from build123d import *

# Parameters (mm, degrees)
BOSS_EXTRUDE1_DEPTH = 2
BOSS_EXTRUDE2_DEPTH = 5
CHAMFER1_SIZE       = 0.2


with BuildPart() as part:
    # Sketch1 → Boss-Extrude1 (new body)
    with BuildSketch(Plane(origin=(0, 0, 0), x_dir=(1, 0, 0), z_dir=(0, 1, 0))):
        with BuildLine():
            Line((60, 26), (30, 26))
            ThreePointArc((30, 26), (26, 30), (30, 34))
            Line((30, 34), (60, 34))
            Line((60, 34), (60, 60))
            Line((60, 60), (0, 60))
            Line((0, 60), (0, 0))
            Line((0, 0), (60, 0))
            Line((60, 0), (60, 26))
        make_face()
    extrude(amount=BOSS_EXTRUDE1_DEPTH)

    # Sketch2 → Boss-Extrude2 (add)
    with BuildSketch(Plane.XZ):
        Polygon((60, -12), (60, -10), (10, -10), (10, -60), (12, -60), (12, -12), align=None)
        Polygon((60, -2), (60, 0), (0, 0), (0, -60), (2, -60), (2, -10), (2, -2), (10, -2), align=None)
    extrude(amount=BOSS_EXTRUDE2_DEPTH)

    # Chamfer1
    chamfer1_edges = [part.edges().sort_by_distance(p)[0] for p in [
        (35, -5, -10),
        (10, -5, -35),
        (11, -5, -60),
        (12, -5, -36),
        (36, -5, -12),
        (60, -5, -11),
        (2, -5, -31),
        (31, -5, -2),
        (60, -5, -1),
        (30, -5, 0),
        (0, -5, -30),
        (1, -5, -60),
    ]]
    chamfer(chamfer1_edges, length=CHAMFER1_SIZE)


solid = part.part
Source: CAD feature listing. Evaluate the final solid. Frame: model axes, mm. A direction names the side the tool comes from. Round coordinates to 2 decimals unless told otherwise and drop trailing zeros. Loops run counter-clockwise (first coordinate to the right, second up) from the corner with the lowest first, then second, coordinate; pieces in that order, holes last. Notation, with made-up numbers: (-31.75, 79) -> (1.25, 79) arc R32 cw to (1.25, 108) -> close; hole circle Ø1 at (20.25, -1). An arc over 180 degrees is marked (long way). Answer as a JSON object with one key per item and string values. Group by question number.
Q1. Contact query for flat-ended pins moving along their axis: P1, Ø24, axis at x = 38.5, z = -34, coming from the -Y side; P2, Ø2.5, axis at x = 42, y = -3, coming from the -Z side; P3, Ø1.4, axis at y = -2.5, z = -40, coming from the +X side. Output: stop coordinate, or through.
Q2. Section query C-C (x = 7.5). Output: boundary loops of the cut face in (y, z), plus the area to 3 significant figures.
Q3. Mould query, pull axis Z, two halves, no side actions, for faces 1 (the flat face through (45, 1, -34)), 2 (the flat face through (60, 0.2, -10.3)), 3 (the flat face through (28, 1, -60)). Classes: pulls with the +Z half, pulls with the -Z half, needs draft (parallel to the pull), parting line crosses it, or undercut.
Q4. Section query D-D (z = -30). Output: boundary loops of the cut face in (x, y).
Q5. Section query B-B (x = 49). Output: boundary loops of the cut face in (y, z).
Q6. Section query A-A (y = -2.5). Output: boundary loops of the cut face in (x, z), plus the area to 3 significant figures.
Q7. Access query for faces 4 (the flat face through (2, -2, -31)), 5 (the flat face through (12, -2, -36)), 6 (the flat face through (31, -2, -2)), 7 (the flat face through (17, -5, -1)), 8 (the flat face through (45, 1, -26)). Directions: +Z, -Z, +X, -X, +Y, -Y. A direction counts if a zero-diameter tool reaches every point of the face in a straight line with its end or side. Return the directions, or none.
Q8. Ray query, line 1 (Z direction, x = 30, y = -1.5); line 2 (X direction, y = -4.5, z = -14); line 3 (Y direction, x = 12.5, z = -31). Return the intervals inside material, ascending. Write a range as from..to.
Completed:
{
 "1": {"P1": "y = 0", "P2": "z = -12", "P3": "x = 12"},
 "2": {"outline": "(-5, -1.8) -> (-4.8, -2) -> (0, -2) -> (0, -60) -> (2, -60) -> (2, 0) -> (-4.8, 0) -> (-5, -0.2) -> close", "area": "130 mm²"},
 "3": {"face 1": "undercut", "face 2": "needs draft", "face 3": "pulls with the -Z half"},
 "4": {"outline": "(0, -4.8) -> (0.2, -5) -> (1.8, -5) -> (2, -4.8) -> (2, 0) -> (10, 0) -> (10, -4.8) -> (10.2, -5) -> (11.8, -5) -> (12, -4.8) -> (12, 0) -> (26, 0) -> (26, 2) -> (0, 2) -> close"},
 "5": {"outline": "(-5, -11.8) -> (-4.8, -12) -> (0, -12) -> (0, -26) -> (2, -26) -> (2, 0) -> (-4.8, 0) -> (-5, -0.2) -> (-5, -1.8) -> (-4.8, -2) -> (0, -2) -> (0, -10) -> (-4.8, -10) -> (-5, -10.2) -> close; (0, -60) -> (2, -60) -> (2, -34) -> (0, -34) -> close"},
 "6": {"outline": "(0, -60) -> (2, -60) -> (2, -2) -> (60, -2) -> (60, 0) -> (0, 0) -> close; (10, -60) -> (12, -60) -> (12, -12) -> (60, -12) -> (60, -10) -> (10, -10) -> close", "area": "432 mm²"},
 "7": {"face 4": "-Z, -Y", "face 5": "-Z, +X, -Y", "face 6": "+X, -Y", "face 7": "+Z, -Z, +X, -X, -Y", "face 8": "+X, +Y, -Y"},
 "8": {"line 1": "-12..-10, -2..0", "line 2": "0..2, 10..12", "line 3": "0..2"}
}
